Check sheet for the modelled part. Datum: model origin and axes. Units: mm. Round coordinates to 2 decimals unless told otherwise and drop trailing zeros. Write each loop counter-clockwise with the first axis right and the second up, starting at its lowest first coordinate (ties: lowest second). Pieces come first, ordered by that corner, then holes. Notation, with made-up numbers: (-27.75, -5.5) -> (-14.75, -5.5) arc R6 cw to (-14.75, 1.5) -> close; hole circle Ø8 at (9, -6). An arc over 180 degrees is marked (long way). Use one line per item in the form item = value. Start each with the question number.
```python
from build123d import *

# Parameters (mm, degrees)
SKETCH1_R           = 52
BOSS_EXTRUDE1_DEPTH = 11
SKETCH2_R           = 7.5
BOSS_EXTRUDE2_DEPTH = 12
SKETCH3_R           = 1.5
BOSS_EXTRUDE3_DEPTH = 17.5
SKETCH4_R           = 3
CUT_EXTRUDE3_DEPTH  = 12


with BuildPart() as part:
    # Sketch1 → Boss-Extrude1 (new, symmetric)
    with BuildSketch(Plane.XY):
        Circle(SKETCH1_R)
    extrude(amount=BOSS_EXTRUDE1_DEPTH, both=True)

    # Sketch2 → Boss-Extrude2 (add)
    with BuildSketch(Plane.XY.offset(11)):
        Circle(SKETCH2_R)
    extrude(amount=BOSS_EXTRUDE2_DEPTH)

    # Sketch3 → Boss-Extrude3 (add)
    with BuildSketch(Plane(origin=(0, 0, 0), x_dir=(1, 0, 0), z_dir=(0, 1, 0))):
        with Locations(Location((0, -17, 0), (0, 0, 90))):
            Circle(SKETCH3_R)
    extrude(amount=BOSS_EXTRUDE3_DEPTH)

    # Sketch4 → Cut-Extrude3 (cut)
    with BuildSketch(Plane(origin=(0, 0, 23), x_dir=(-1, 0, 0), z_dir=(0, 0, -1))):
        Circle(SKETCH4_R)
    extrude(amount=CUT_EXTRUDE3_DEPTH, mode=Mode.SUBTRACT)


solid = part.part
```
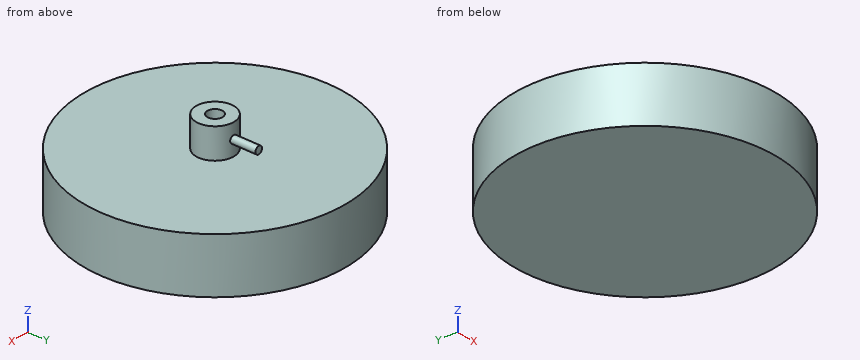
1. Scan lines: probe 1 along Y at (x, z) = (0, 16); probe 2 along Y at (x, z) = (0, 15); probe 3 along Z at (x, y) = (-34, 19.5). Record each from-to range of solid material in increasing order.
2. Sectioned sample at D-D (y = 10.5). Enter the section's corners in (x, z).
3. Depth check by flat-ended pin: pin 1 (5 mm diameter, centred on x = 7, y = 11, fed in from +Z); pin 2 (2 mm diameter, centred on y = 27.5, z = 0, fed in from -X); pin 3 (3 mm diameter, centred on x = 24, z = -5, fed in from -Y). Enter the tip coordinate at first touch or a pass-through.
4. Sectioned sample at C-C (x = 0). Enter the section's corners in (y, z), and give its area (3 significant figures).
5. Sectioned sample at A-A (y = 0). Enter the section's corners in (x, z).
6. Sectioned sample at B-B (z = 17). Enter the section's corners in (x, y), and give its area (3 significant figures).
Returned:
q1.probe_1 = -7.5 to -3, 3 to 17.5
q1.probe_2 = -7.5 to -3, 3 to 7.5
q1.probe_3 = -11 to 11
q2.outline = (-50.93, -11) -> (50.93, -11) -> (50.93, 11) -> (-50.93, 11) -> close; circle Ø3 at (0, 17)
q3.pin_1 = 11
q3.pin_2 = -44.74
q3.pin_3 = -46.88
q4.outline = (-52, -11) -> (52, -11) -> (52, 11) -> (7.5, 11) -> (7.5, 15.5) -> (17.5, 15.5) -> (17.5, 18.5) -> (7.5, 18.5) -> (7.5, 23) -> (3, 23) -> (3, 11) -> (-3, 11) -> (-3, 23) -> (-7.5, 23) -> (-7.5, 11) -> (-52, 11) -> close
q4.area = 2,430 mm^2
q5.outline = (-52, -11) -> (52, -11) -> (52, 11) -> (7.5, 11) -> (7.5, 23) -> (3, 23) -> (3, 11) -> (-3, 11) -> (-3, 23) -> (-7.5, 23) -> (-7.5, 11) -> (-52, 11) -> close
q6.outline = (-1.5, 7.35) arc R7.5 ccw (long way) to (1.5, 7.35) -> (1.5, 17.5) -> (-1.5, 17.5) -> close; hole circle Ø6 at (0, 0)
q6.area = 179 mm^2
